Geometry check sheet. Reference: the model listing, model coordinates, mm. A direction names the side the tool comes from. Round coordinates to 2 decimals unless told otherwise and drop trailing zeros. Write each loop counter-clockwise with the first axis right and the second up, starting at its lowest first coordinate (ties: lowest second). Pieces come first, ordered by that corner, then holes. Notation, with made-up numbers: M -2.75,65 L 2.25,65 A16 ccw 2.25,86 Z; hole C -1,55 d11. An arc over 180 degrees is marked long. Put each result on its own line as item: value. Start each with the question number.
(1) Section check C-C on x = -10.5. Record the cut outline in (y, z), then the cut area to 3 significant figures.
(2) Tool access check on faces 1 (the flat face through (11.5, 6, 0)), 2 (the flat face through (-4.4, -8, 0)), 3 (the flat face through (6.5, 6, -13)), 4 (the flat face through (6.5, 6, 13)). Record the directions out of +Z, -Z, +X, -X, +Y, -Y that give a thin tool (end or side, any length) a straight path to the whole face; none if there is none.
(3) Material ranges on probe 1 along Z at (x, y) = (2.5, -4.5); probe 2 along Y at (x, z) = (0, -21); probe 3 along X at (y, z) = (0, -21.5), recorded low to high.
(4) Section check A-A on y = 0. Record the cut outline in (x, z).
(5) Gauge pin test, flat ends, axial feed: pin 1 (4.5 mm diameter, centred on y = 5.5, z = 9.5, fed in from -X); pin 2 (1.5 mm diameter, centred on x = 8.5, y = 6, fed in from +Z); pin 3 (3 mm diameter, centred on y = 5.5, z = 14.5, fed in from -X). Record the tip position at first contact, or that the pin passes through.
(6) Section check B-B on y = -6.75. Record the cut outline in (x, z).
(7) Mould release check, pull along Z, two halves, no side actions. Record for faces 5 (the flat face through (-2, -5.5, 0)), 6 (the cylindrical face through (3.252, 6.128, 5.037)), 7 (the flat face through (7.5, 6, -7)): pulls with the +Z half, pulls with the -Z half, needs draft (parallel to the pull), parting line crosses it, or undercut.
from build123d import *

# Parameters (mm, degrees)
BOSS_EXTRUDE1_DEPTH    = 9.15
BOSS_EXTRUDE2_DEPTH    = 3
BOSS_EXTRUDE3_START    = -23
SKETCH4_R              = 5.5
BOSS_EXTRUDE3_DEPTH    = 23.75
MOVE_START             = 3.6
MOVE_FACE1_OUTLINE_W   = 12.5
MOVE_FACE1_OUTLINE_H   = 46
MOVE_FACE1_DEPTH       = 0.5
MOVE_START_2           = -1.4
MOVE_FACE2_OUTLINE_W   = 10.5
MOVE_FACE2_OUTLINE_H   = 46
MOVE_FACE2_DEPTH       = 2
SKETCH7_R              = 5.5
CUT_EXTRUDE1_DEPTH     = 7.5
HOLE2_START            = -23.75
HOLE2_OUTLINE_R        = 3
HOLE2_DEPTH            = 47.5
BOSS_EXTRUDE4_REACH    = 35.801
SKETCH10_W             = 4
SKETCH10_H             = 11.5
FILLET1_R              = 2.5
FILLET3_R              = 0.5
CUT_EXTRUDE2_DEPTH     = 4
SKETCH12_W             = 6
SKETCH12_H             = 2
BOSS_EXTRUDE5_DEPTH    = 4
FILLET2_R              = 1
LPATTERN2_COUNT        = 3
LPATTERN2_PITCH        = 4.5
FILLET2_OF_LPATTERN2_R = 1
SKETCH13_R             = 3.5
BOSS_EXTRUDE13_DEPTH   = 4
MIRROR1_START          = 7.5
MIRROR1_DEPTH          = 4
MIRROR1_START_2        = 9.15
MIRROR1_2_OUTLINE_R    = 3
MIRROR1_2_DEPTH        = 7.5


# Read off the part's stored shape, not the designer's step: Move Face1, Move Face2, Hole2, Mirror1
# Some blends are built 0.0001 mm under size
with BuildPart() as part:
    # Sketch1 → Boss-Extrude1 (new, symmetric)
    with BuildSketch(Plane.XY):
        with BuildLine():
            Line((-4.4, -5.5), (0, -5.5))
            ThreePointArc((0, -5.5), (5.5, 0), (0, 5.5))
            Line((0, 5.5), (-7, 5.5))
            Line((-7, 5.5), (-7, 8.1))
            Line((-7, 8.1), (-12.563102278, 8.1))
            Line((-12.563102278, 8.1), (-15, 0.6))
            Line((-15, 0.6), (-15, -8.830934004))
            Line((-15, -8.830934004), (-4.4, -10.7))
            Line((-4.4, -10.7), (-4.4, -5.5))
        make_face()
    extrude(amount=BOSS_EXTRUDE1_DEPTH, both=True)

    # Sketch3 → Boss-Extrude2 (add)
    with BuildSketch(Plane(origin=(0, 0.6, 0), x_dir=(0, 0, -1), z_dir=(0, 1, 0))):
        Polygon((17, 9.5), (-17, 9.5), (-23, 6.035898385), (-23, -14.5), (23, -14.5), (23, 6.035898385), align=None)
    extrude(amount=BOSS_EXTRUDE2_DEPTH)

    # Sketch4 → Boss-Extrude3 (add, symmetric)
    with BuildSketch(Plane(origin=(0, 0, -23), x_dir=(-1, 0, 0), z_dir=(0, 0, -1)).offset(BOSS_EXTRUDE3_START)):
        with Locations(Location((0, 0, 0), (0, 0, 180))):
            Circle(SKETCH4_R)
    extrude(amount=BOSS_EXTRUDE3_DEPTH, both=True)

    # Move Face1 outline → Move Face1 (add)
    with BuildSketch(Plane(origin=(0, 0, 0), x_dir=(1, 0, 0), z_dir=(0, 1, 0)).offset(MOVE_START)):
        with Locations((8.25, 0)):
            Rectangle(MOVE_FACE1_OUTLINE_W, MOVE_FACE1_OUTLINE_H)
    extrude(amount=MOVE_FACE1_DEPTH)

    # Move Face2 outline → Move Face2 (add)
    with BuildSketch(Plane(origin=(0, 0, 0), x_dir=(1, 0, 0), z_dir=(0, 1, 0)).offset(MOVE_START_2)):
        with Locations((9.25, 0)):
            Rectangle(MOVE_FACE2_OUTLINE_W, MOVE_FACE2_OUTLINE_H)
    extrude(amount=MOVE_FACE2_DEPTH)

    # Sketch7 → Cut-Extrude1 (cut)
    with BuildSketch(Plane(origin=(0, 0, -9.15), x_dir=(-1, 0, 0), z_dir=(0, 0, -1))):
        with Locations(Location((0, 0, 0), (0, 0, 6.262913126))):
            Circle(SKETCH7_R)
    extrude(amount=CUT_EXTRUDE1_DEPTH, mode=Mode.SUBTRACT)

    # Hole2 outline → Hole2 (cut)
    with BuildSketch(Plane.XY.offset(HOLE2_START)):
        Circle(HOLE2_OUTLINE_R)
    extrude(amount=HOLE2_DEPTH, mode=Mode.SUBTRACT)

    # Boss-Extrude4: up to this face of the body (flat: up to its plane)
    boss_extrude4_end = Plane(part.part.faces().sort_by_distance((9.083030278, 4.1, 0))[0])
    # Sketch10 → Boss-Extrude4 (add, up to the picked face)
    with BuildSketch(Plane(origin=(0, 8.1, 0), x_dir=(1, 0, 0), z_dir=(0, 1, 0)), mode=Mode.PRIVATE) as boss_extrude4_sk1:
        with BuildLine():
            Line((12.5, -19), (12.5, 19))
            ThreePointArc((12.5, 19), (9.5, 22), (6.5, 19))
            Line((6.5, 19), (6.5, 5.75))
            Line((6.5, 5.75), (10.5, 5.75))
            Line((10.5, 5.75), (10.5, -5.75))
            Line((10.5, -5.75), (6.5, -5.75))
            Line((6.5, -5.75), (6.5, -19))
            ThreePointArc((6.5, -19), (9.5, -22), (12.5, -19))
        make_face()
    boss_extrude4_tool1 = split(extrude(boss_extrude4_sk1.sketch, amount=-BOSS_EXTRUDE4_REACH, mode=Mode.PRIVATE), bisect_by=boss_extrude4_end, keep=Keep.BOTH, mode=Mode.PRIVATE)
    # Sketch10 → Boss-Extrude4 (add, up to the picked face)
    with BuildSketch(Plane(origin=(0, 8.1, 0), x_dir=(1, 0, 0), z_dir=(0, 1, 0)), mode=Mode.PRIVATE) as boss_extrude4_sk2:
        with Locations((8.5, 0)):
            Rectangle(SKETCH10_W, SKETCH10_H)
    boss_extrude4_tool2 = split(extrude(boss_extrude4_sk2.sketch, amount=-BOSS_EXTRUDE4_REACH, mode=Mode.PRIVATE), bisect_by=boss_extrude4_end, keep=Keep.BOTH, mode=Mode.PRIVATE)
    # Sketch10 → Boss-Extrude4 (add, up to the picked face)
    with BuildSketch(Plane(origin=(0, 8.1, 0), x_dir=(1, 0, 0), z_dir=(0, 1, 0)), mode=Mode.PRIVATE) as boss_extrude4_sk3:
        with Locations((4.5, 0)):
            Rectangle(SKETCH10_W, SKETCH10_H)
    boss_extrude4_tool3 = split(extrude(boss_extrude4_sk3.sketch, amount=-BOSS_EXTRUDE4_REACH, mode=Mode.PRIVATE), bisect_by=boss_extrude4_end, keep=Keep.BOTH, mode=Mode.PRIVATE)
    add(boss_extrude4_tool1.solids().sort_by(Axis((12.055928, 8.1, 0), (0, -1, 0)))[0])
    add(boss_extrude4_tool2.solids().sort_by(Axis((8.5, 8.1, 0), (0, -1, 0)))[0])
    add(boss_extrude4_tool3.solids().sort_by(Axis((4.5, 8.1, 0), (0, -1, 0)))[0])

    # Fillet1
    # the kernel refuses this fillet: 2.5 mm, written as the material it takes off along each edge
    with BuildSketch(Plane(origin=(2.5, 14.35, -5.75), x_dir=(1, 0, 0), z_dir=(0, -1, 0))) as fillet1_piece_1_section:
        with BuildLine():
            CenterArc((FILLET1_R, FILLET1_R), FILLET1_R, 180, 90)
            Line((0, FILLET1_R), (0, 0))
            Line((0, 0), (FILLET1_R, 0))
        make_face()
    fillet1_piece_1 = extrude(amount=15.701020514, mode=Mode.PRIVATE)
    fillet1_piece_1 = fillet1_piece_1 - Plane(origin=(0, 0, -5.193529693), x_dir=(0, -1, 0), z_dir=(0, 0, 1)) * Cylinder(5.5, 42, mode=Mode.PRIVATE)
    fillet1_piece_1 = split(fillet1_piece_1, bisect_by=Plane(origin=(3.08088975, 4.1, -5.193529693), z_dir=(0, 1, 0)), keep=Keep.TOP, mode=Mode.PRIVATE)
    add(fillet1_piece_1, mode=Mode.SUBTRACT)
    with BuildSketch(Plane(origin=(2.5, 14.35, 5.75), x_dir=(0, 0, -1), z_dir=(0, -1, 0))) as fillet1_piece_2_section:
        with BuildLine():
            CenterArc((FILLET1_R, FILLET1_R), FILLET1_R, 180, 90)
            Line((0, FILLET1_R), (0, 0))
            Line((0, 0), (FILLET1_R, 0))
        make_face()
    fillet1_piece_2 = extrude(amount=15.701020514, mode=Mode.PRIVATE)
    fillet1_piece_2 = fillet1_piece_2 - Plane(origin=(0, 0, 5.193529696), x_dir=(0, -1, 0), z_dir=(0, 0, 1)) * Cylinder(5.5, 42, mode=Mode.PRIVATE)
    fillet1_piece_2 = split(fillet1_piece_2, bisect_by=Plane(origin=(3.080889748, 4.1, 5.193529696), z_dir=(0, 1, 0)), keep=Keep.TOP, mode=Mode.PRIVATE)
    add(fillet1_piece_2, mode=Mode.SUBTRACT)

    # Fillet3
    fillet3_edges = [part.edges().sort_by_distance(p)[0] for p in [
        (6.5, 6.1, 5.75),
        (6.5, 6.1, -5.75),
    ]]
    fillet(fillet3_edges, radius=FILLET3_R)

    # Sketch11 → Cut-Extrude2 (cut)
    with BuildSketch(Plane(origin=(0, 8.1, 0), x_dir=(1, 0, 0), z_dir=(0, 1, 0))):
        with BuildLine():
            Line((6, 4.75), (5, 4.75))
            ThreePointArc((5, 4.75), (3.939339828, 4.310660172), (3.5, 3.25))
            Line((3.5, 3.25), (3.5, -3.25))
            ThreePointArc((3.5, -3.25), (3.939339828, -4.310660172), (5, -4.75))
            Line((5, -4.75), (6, -4.75))
            ThreePointArc((6, -4.75), (7.060660172, -5.189339828), (7.5, -6.25))
            Line((7.5, -6.25), (7.5, -19))
            ThreePointArc((7.5, -19), (9.5, -21), (11.5, -19))
            Line((11.5, -19), (11.5, 19))
            ThreePointArc((11.5, 19), (9.5, 21), (7.5, 19))
            Line((7.5, 19), (7.5, 6.25))
            ThreePointArc((7.5, 6.25), (7.060660172, 5.189339828), (6, 4.75))
        make_face()
    extrude(amount=-CUT_EXTRUDE2_DEPTH, mode=Mode.SUBTRACT)

    # Sketch12 → Boss-Extrude5 (add)
    with BuildSketch(Plane(origin=(0, 4.1, 0), x_dir=(1, 0, 0), z_dir=(0, 1, 0))):
        with Locations((9.5, 17.25)):
            Rectangle(SKETCH12_W, SKETCH12_H)
    boss_extrude5 = extrude(amount=BOSS_EXTRUDE5_DEPTH)

    # Fillet2
    fillet2_edges = [part.edges().sort_by_distance(p)[0] for p in [
        (9.5, 8.1, -18.25),
        (9.5, 8.1, -16.25),
    ]]
    fillet(fillet2_edges, radius=FILLET2_R - 0.0001)  # a hair under: the kernel refuses the full size

    # LPattern2: Boss-Extrude5 ×3
    with Locations(*[(0, 0, i * LPATTERN2_PITCH) for i in range(1, LPATTERN2_COUNT)]):
        add(boss_extrude5)

    # Fillet2 of LPattern2
    fillet2_of_lpattern2_edges = [part.edges().sort_by_distance(p)[0] for p in [
        (9.5, 8.1, -13.75),
        (9.5, 8.1, -11.75),
        (9.5, 8.1, -9.25),
        (9.5, 8.1, -7.25),
    ]]
    fillet(fillet2_of_lpattern2_edges, radius=FILLET2_OF_LPATTERN2_R - 0.0001)  # a hair under: the kernel refuses the full size

    # Sketch13 → Boss-Extrude13 (add)
    with BuildSketch(Plane(origin=(0, 4.1, 0), x_dir=(1, 0, 0), z_dir=(0, 1, 0))):
        with Locations(Location((7.00001, 0, 0), (0, 0, 270))):
            Circle(SKETCH13_R)
    extrude(amount=BOSS_EXTRUDE13_DEPTH)

    # Mirror1 outline → Mirror1 (add)
    with BuildSketch(Plane.YZ.offset(MIRROR1_START)):
        with BuildLine():
            ThreePointArc((8.1, 17.25), (7.807106781, 17.957106781), (7.1, 18.25))
            Line((7.1, 18.25), (4.1, 18.25))
            Line((4.1, 18.25), (4.1, 16.25))
            Line((4.1, 16.25), (7.1, 16.25))
            ThreePointArc((7.1, 16.25), (7.807106781, 16.542893219), (8.1, 17.25))
        make_face()
        with BuildLine():
            Line((7.1, 9.25), (4.1, 9.25))
            Line((4.1, 9.25), (4.1, 7.25))
            Line((4.1, 7.25), (7.1, 7.25))
            ThreePointArc((7.1, 7.25), (7.807106781, 7.542893219), (8.1, 8.25))
            ThreePointArc((8.1, 8.25), (7.807106781, 8.957106781), (7.1, 9.25))
        make_face()
        with BuildLine():
            Line((7.1, 13.75), (4.1, 13.75))
            Line((4.1, 13.75), (4.1, 11.75))
            Line((4.1, 11.75), (7.1, 11.75))
            ThreePointArc((7.1, 11.75), (7.807106781, 12.042893219), (8.1, 12.75))
            ThreePointArc((8.1, 12.75), (7.807106781, 13.457106781), (7.1, 13.75))
        make_face()
    extrude(amount=MIRROR1_DEPTH)

    # Mirror1 2 outline → Mirror1 2 (cut)
    with BuildSketch(Plane.XY.offset(MIRROR1_START_2)):
        with BuildLine():
            ThreePointArc((5.318834459, -1.4), (5.267312845, 1.582850401), (3.666060556, 4.1))
            ThreePointArc((3.666060556, 4.1), (-0.350758821, 5.4888039), (-4.158124577, 3.6))
            ThreePointArc((-4.158124577, 3.6), (-5.040991658, 2.199637039), (-5.467174773, 0.6))
            ThreePointArc((-5.467174773, 0.6), (-1.002746834, -5.407818302), (5.318834459, -1.4))
        make_face()
        Circle(MIRROR1_2_OUTLINE_R, mode=Mode.SUBTRACT)
    extrude(amount=MIRROR1_2_DEPTH, mode=Mode.SUBTRACT)


solid = part.part
Answers follow:
1. outline: M -9.62,-9.15 L 8.1,-9.15 L 8.1,9.15 L -9.62,9.15 Z
1. area: 324 mm^2
2. face 1: +Y
2. face 2: +Z, -Z, +X, -Y
2. face 3: -Z, +Y
2. face 4: +Z, +Y
3. probe 1: z = -23.75 to -16.65, -9.15 to 9.15, 16.65 to 23.75
3. probe 2: y = -5.5 to -3, 3 to 5.5
3. probe 3: x = -5.5 to -3, 3 to 14.5
4. outline: M -15,-9.15 L -3,-9.15 L -3,9.15 L -15,9.15 Z; M -5.5,-23.75 L -3,-23.75 L -3,-16.65 L -5.5,-16.65 Z; M -5.5,16.65 L -3,16.65 L -3,23.75 L -5.5,23.75 Z; M 3,-23.75 L 5.5,-23.75 L 5.5,-23 L 14.5,-23 L 14.5,23 L 5.5,23 L 5.5,23.75 L 3,23.75 L 3,16.65 L 5.5,16.65 L 5.5,9.15 L 3,9.15 L 3,-9.15 L 5.5,-9.15 L 5.5,-16.65 L 3,-16.65 Z
5. pin 1: stops at x = -14.13
5. pin 2: stops at z = 21.99
5. pin 3: stops at x = 3.67
6. outline: M -15,-9.15 L -4.4,-9.15 L -4.4,9.15 L -15,9.15 Z
7. face 5: needs draft
7. face 6: pulls with the +Z half
7. face 7: undercut
